from build123d import *

# Parameters (mm, degrees)
SKETCH2_W           = 177.8
SKETCH2_H           = 177.8
BOSS_EXTRUDE2_DEPTH = 12.7
SKETCH2_2_W         = 177.8
SKETCH2_2_H         = 177.8
BOSS_EXTRUDE3_DEPTH = 3
SKETCH3_W           = 38.1
SKETCH3_H           = 88.9
BOSS_EXTRUDE4_DEPTH = 104.6
BOSS_EXTRUDE5_DEPTH = 53.8


with BuildPart() as part:
    # Sketch2 → Boss-Extrude2 (new body)
    with BuildSketch(Plane(origin=(0, 0, 0), x_dir=(1, 0, 0), z_dir=(0, 1, 0))):
        Rectangle(SKETCH2_W, SKETCH2_H)
    extrude(amount=BOSS_EXTRUDE2_DEPTH)

    # Sketch2<2> → Boss-Extrude3 (add)
    with BuildSketch(Plane(origin=(0, 0, 0), x_dir=(1, 0, 0), z_dir=(0, 1, 0))):
        Rectangle(SKETCH2_2_W, SKETCH2_2_H)
    extrude(amount=-BOSS_EXTRUDE3_DEPTH)

    # Sketch3 → Boss-Extrude4 (add)
    with BuildSketch(Plane.XZ.offset(3)):
        Polygon((-25.475339684, -50.8), (-63.5, -17.113723747), (-29.813723747, 20.91093657), (8.21093657, -12.775339684), align=None)
        with Locations((44.45, 6.35)):
            Rectangle(SKETCH3_W, SKETCH3_H)
    extrude(amount=BOSS_EXTRUDE4_DEPTH)

    # Sketch4 → Boss-Extrude5 (add)
    with BuildSketch(Plane.XZ.offset(107.6)):
        Polygon((-25.475339684, -50.8), (44.89207381, -21.561889285), (25.4, 25.349719711), (-44.967413494, -3.888391004), align=None)
    extrude(amount=BOSS_EXTRUDE5_DEPTH)


solid = part.part
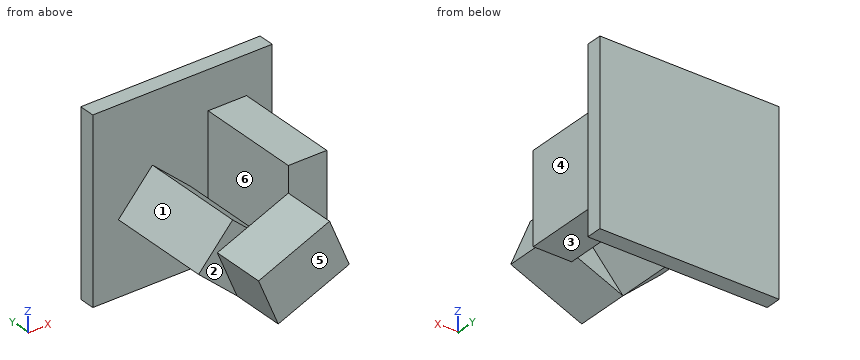
Read the model definition and answer for the solid it produces. Units are mm, in the model's axes. Face numbers are marked on the shaded views. A direction names the side the tool comes from. Round coordinates to 2 decimals unless told otherwise and drop trailing zeros. Order: outer loops, then holes, each group sorted by start corner. A loop starts at its lowest first (then second) coordinate and runs counter-clockwise, first axis right, second up.
1) The mould has two halves that part along Y. Classify the marked faces 4, 5 and 6: released by +Y, released by -Y, zero draft, split by the parting line, or undercut.
2) The part is cut by section C-C on y = -124. Write down the section's boundary in (x, z).
3) The part is cut by section A-A on y = -12. Write down the section's boundary in (x, z).
4) Straight lines are drawn through the part: L1, parallel to Y at x = -2.5, z = -2; L2, parallel to Y at x = -41, z = 70; L3, parallel to X at y = -57, z = -12. For each, find the intervals that lie inside material, in ascending order.
5) The part is cut by section D-D on z = 78. Write down the section's boundary in (x, y).
6) For the marked faces 1, 2 and 3, determine the directions among +Z, -Z, +X, -X, +Y, -Y from which every point of the face is accessible in a straight line to the end or side of a thin tool.
7) Flat-ended cylindrical pins translate along their axes: pin 1 (1.5 mm diameter, centred on x = -40.5, y = -125, fed in from -Z); pin 2 (6 mm diameter, centred on x = -57.5, y = -48, fed in from -Z); pin 3 (2 mm diameter, centred on y = -88.5, z = -2.5, fed in from -X). Find the tip coordinate at first contact, or state that the pin passes through.
8) The part is cut by section B-B on x = 49. Write down the section's boundary in (y, z).
Resolved:
1. face 4: zero draft
1. face 5: released by -Y
1. face 6: undercut
2. outline: (-44.97, -3.89) - (-25.48, -50.8) - (44.89, -21.56) - (25.4, 25.35) - close
3. outline: (-63.5, -17.11) - (-25.48, -50.8) - (8.21, -12.78) - (-29.81, 20.91) - close; (25.4, -38.1) - (63.5, -38.1) - (63.5, 50.8) - (25.4, 50.8) - close
4. L1: y = -161.4 to -107.6, -3 to 12.7
4. L2: y = -3 to 12.7
4. L3: x = -58.97 to 7.34, 25.4 to 63.5
5. outline: (-88.9, -3) - (88.9, -3) - (88.9, 12.7) - (-88.9, 12.7) - close
6. face 1: +Z, -X, -Y
6. face 2: -X, -Y
6. face 3: -Z, +X, -Y
7. pin 1: stops at z = -16.45
7. pin 2: stops at z = -25.09
7. pin 3: stops at x = -51.44
8. outline: (-107.6, -38.1) - (-3, -38.1) - (-3, -88.9) - (12.7, -88.9) - (12.7, 88.9) - (-3, 88.9) - (-3, 50.8) - (-107.6, 50.8) - close
